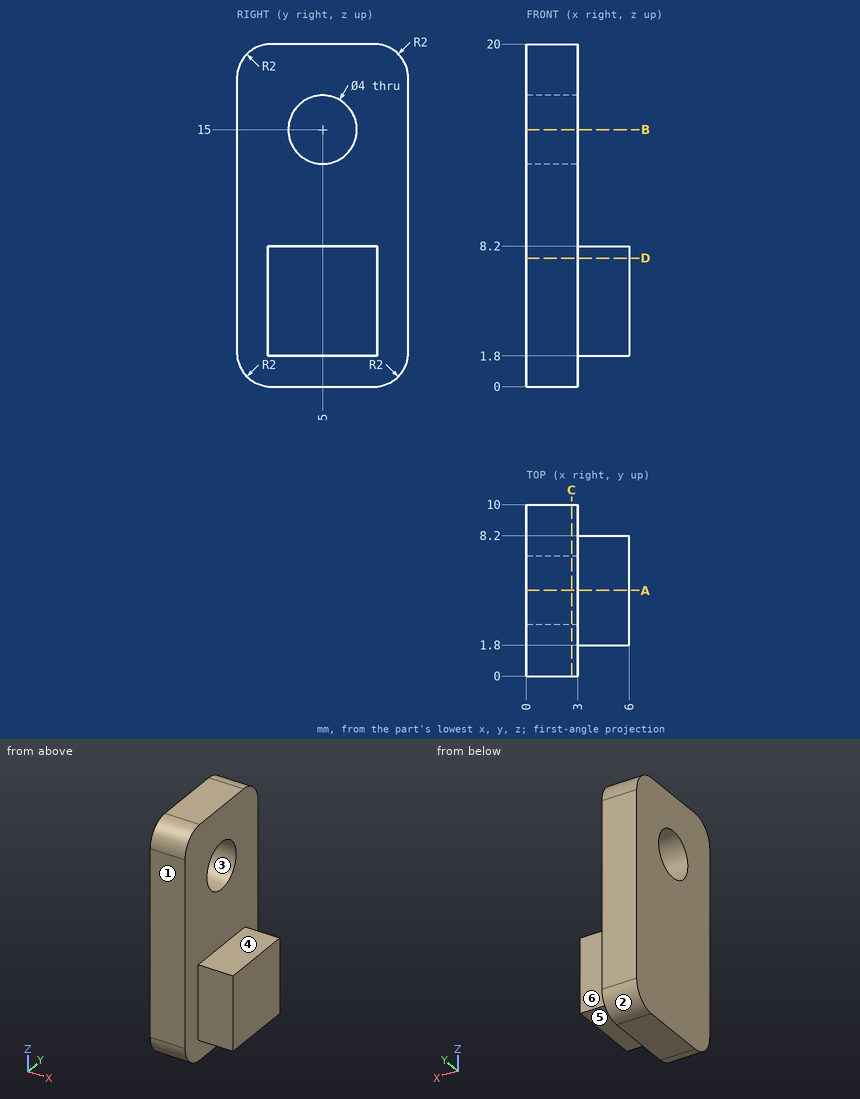
Geometry check sheet. Reference: drawing and pictorial views, mm from the part's lowest x, y, z. A direction names the side the tool comes from. Round coordinates to 2 decimals unless told otherwise and drop trailing zeros. Write each loop counter-clockwise with the first axis right and the second up, starting at its lowest first coordinate (ties: lowest second). Pieces come first, ordered by that corner, then holes.
1. Section check B-B on z = 15. Enter the section's corners in (x, y), plus the area to 3 significant figures.
2. Section check A-A on y = 5. Enter the section's corners in (x, z), plus the area to 3 significant figures.
3. Scan lines: L1, parallel to Y at x = 1.05, z = 15; L2, parallel to Z at x = 3.25, y = 7.25; L3, parallel to X at y = 1, z = 12. Record each from-to range of solid material in increasing order.
4. Draft check along Y on the marked faces 1, 2 and 3. Enter one of: +Y half, -Y half, draft (parallel to the pull), parting line (faces both ways), or undercut.
5. Gauge pin test, flat ends, axial feed: P1, Ø1.5, axis at x = 4.5, z = 5.5, coming from the +Y side; P2, Ø0.9, axis at x = 4, y = 5.5, coming from the +Z side; P3, Ø1.5, axis at x = 4, y = 5, coming from the -Z side. Record the tip position at first contact, or that the pin passes through.
6. Section check D-D on z = 7.5. Enter the section's corners in (x, y).
7. Access from +Z, -Z, +X, -X, +Y, -Y to the whole of each face (thin tool, end or side, straight path). Record for the marked faces 4, 5 and 6.
8. Section check C-C on x = 2.65. Enter the section's corners in (y, z).
Answer:
1. outline: (0, 0) - (3, 0) - (3, 3) - (0, 3) - close; (0, 7) - (3, 7) - (3, 10) - (0, 10) - close
1. area: 18.0 mm2
2. outline: (0, 0) - (3, 0) - (3, 1.8) - (6, 1.8) - (6, 8.2) - (3, 8.2) - (3, 13) - (0, 13) - close; (0, 17) - (3, 17) - (3, 20) - (0, 20) - close
2. area: 67.2 mm2
3. L1: y = 0 to 3, 7 to 10
3. L2: z = 1.8 to 8.2
3. L3: x = 0 to 3
4. face 1: -Y half
4. face 2: +Y half
4. face 3: undercut
5. P1: stops at y = 8.2
5. P2: stops at z = 8.2
5. P3: stops at z = 1.8
6. outline: (0, 0) - (3, 0) - (3, 1.8) - (6, 1.8) - (6, 8.2) - (3, 8.2) - (3, 10) - (0, 10) - close
7. face 4: +Z, +X, +Y, -Y
7. face 5: -Z, +X, +Y, -Y
7. face 6: +Z, -Z, +X, +Y
8. outline: (0, 2) arc R2 ccw to (2, 0) - (8, 0) arc R2 ccw to (10, 2) - (10, 18) arc R2 ccw to (8, 20) - (2, 20) arc R2 ccw to (0, 18) - close; hole circle Ø4 at (5, 15)
